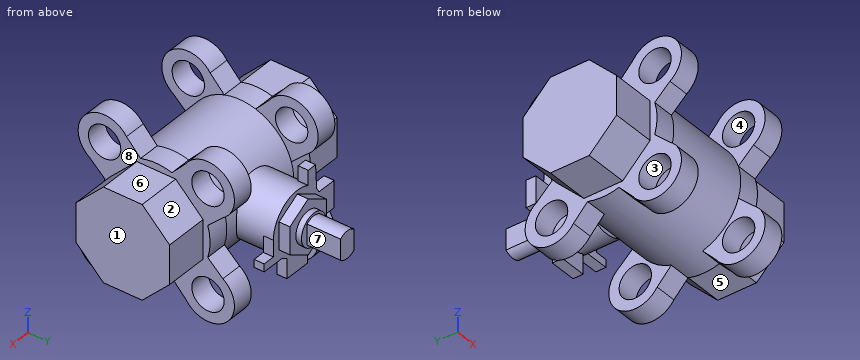
from build123d import *

# Parameters (mm, degrees)
SKETCH1_R            = 4.73075
BOSS_EXTRUDE2_DEPTH  = 6.35
BOSS_EXTRUDE3_DEPTH  = 12.7
SKETCH3_R            = 15.7226
BOSS_EXTRUDE4_DEPTH  = 25.4
SKETCH4_R            = 4.73075
BOSS_EXTRUDE5_DEPTH  = 6.35
BOSS_EXTRUDE6_DEPTH  = 12.7
SKETCH6_R            = 9.0805
BOSS_EXTRUDE8_DEPTH  = 12.8778
SKETCH8_W            = 7.8486
SKETCH8_H            = 8.0772
SKETCH8_W_2          = 8.0772
SKETCH8_H_2          = 7.8486
BOSS_EXTRUDE9_DEPTH  = 2.9464
BOSS_EXTRUDE10_DEPTH = 2.9464
BOSS_EXTRUDE11_DEPTH = 3.175
SKETCH12_R           = 4.6736
BOSS_EXTRUDE12_DEPTH = 1.651
BOSS_EXTRUDE13_DEPTH = 9.779


with BuildPart() as part:
    # Sketch1 → Boss-Extrude2 (new body)
    with BuildSketch(Plane(origin=(0, 0, 0), x_dir=(0, 0, -1), z_dir=(1, 0, 0))):
        with BuildLine():
            Line((-19.4818, 8.715375788), (-15.0368, 4.592907197))
            ThreePointArc((-15.0368, 4.592907197), (-15.7226, 0), (-15.0368, -4.592907197))
            Line((-15.0368, -4.592907197), (-19.4818, -8.715375788))
            ThreePointArc((-19.4818, -8.715375788), (-20.590956234, -20.590956234), (-8.715375788, -19.4818))
            Line((-8.715375788, -19.4818), (-4.592907197, -15.0368))
            ThreePointArc((-4.592907197, -15.0368), (0, -15.7226), (4.592907197, -15.0368))
            Line((4.592907197, -15.0368), (8.715375788, -19.4818))
            ThreePointArc((8.715375788, -19.4818), (20.590956234, -20.590956234), (19.4818, -8.715375788))
            Line((19.4818, -8.715375788), (15.0368, -4.592907197))
            ThreePointArc((15.0368, -4.592907197), (15.7226, 0), (15.0368, 4.592907197))
            Line((15.0368, 4.592907197), (19.4818, 8.715375788))
            ThreePointArc((19.4818, 8.715375788), (20.590956234, 20.590956234), (8.715375788, 19.4818))
            Line((8.715375788, 19.4818), (4.592907197, 15.0368))
            ThreePointArc((4.592907197, 15.0368), (0, 15.7226), (-4.592907197, 15.0368))
            Line((-4.592907197, 15.0368), (-8.715375788, 19.4818))
            ThreePointArc((-8.715375788, 19.4818), (-20.590956234, 20.590956234), (-19.4818, 8.715375788))
        make_face()
        with Locations((-15.113, 15.113)):
            Circle(SKETCH1_R, mode=Mode.SUBTRACT)
        with Locations((15.113, 15.113)):
            Circle(SKETCH1_R, mode=Mode.SUBTRACT)
        with Locations((15.113, -15.113)):
            Circle(SKETCH1_R, mode=Mode.SUBTRACT)
        with Locations((-15.113, -15.113)):
            Circle(SKETCH1_R, mode=Mode.SUBTRACT)
    extrude(amount=BOSS_EXTRUDE2_DEPTH)

    # Sketch2 → Boss-Extrude3 (add)
    with BuildSketch(Plane.ZY):
        Polygon((13.680992893, 5.666852803), (13.680992893, -5.666852803), (5.666852803, -13.680992893), (-5.666852803, -13.680992893), (-13.680992893, -5.666852803), (-13.680992893, 5.666852803), (-5.666852803, 13.680992893), (5.666852803, 13.680992893), align=None)
    extrude(amount=BOSS_EXTRUDE3_DEPTH)

    # Sketch3 → Boss-Extrude4 (add)
    with BuildSketch(Plane(origin=(6.35, 0, 0), x_dir=(0, 0, -1), z_dir=(1, 0, 0))):
        Circle(SKETCH3_R)
    extrude(amount=BOSS_EXTRUDE4_DEPTH)

    # Sketch4 → Boss-Extrude5 (add)
    with BuildSketch(Plane(origin=(31.75, 0, 0), x_dir=(0, 0, -1), z_dir=(1, 0, 0))):
        with BuildLine():
            Line((-19.4818, 8.715375788), (-15.0368, 4.592907197))
            ThreePointArc((-15.0368, 4.592907197), (-15.7226, 0), (-15.0368, -4.592907197))
            Line((-15.0368, -4.592907197), (-19.4818, -8.715375788))
            ThreePointArc((-19.4818, -8.715375788), (-20.590956234, -20.590956234), (-8.715375788, -19.4818))
            Line((-8.715375788, -19.4818), (-4.592907197, -15.0368))
            ThreePointArc((-4.592907197, -15.0368), (0, -15.7226), (4.592907197, -15.0368))
            Line((4.592907197, -15.0368), (8.715375788, -19.4818))
            ThreePointArc((8.715375788, -19.4818), (20.590956234, -20.590956234), (19.4818, -8.715375788))
            Line((19.4818, -8.715375788), (15.0368, -4.592907197))
            ThreePointArc((15.0368, -4.592907197), (15.7226, 0), (15.0368, 4.592907197))
            Line((15.0368, 4.592907197), (19.4818, 8.715375788))
            ThreePointArc((19.4818, 8.715375788), (20.590956234, 20.590956234), (8.715375788, 19.4818))
            Line((8.715375788, 19.4818), (4.592907197, 15.0368))
            ThreePointArc((4.592907197, 15.0368), (0, 15.7226), (-4.592907197, 15.0368))
            Line((-4.592907197, 15.0368), (-8.715375788, 19.4818))
            ThreePointArc((-8.715375788, 19.4818), (-20.590956234, 20.590956234), (-19.4818, 8.715375788))
        make_face()
        with Locations((-15.113, 15.113)):
            Circle(SKETCH4_R, mode=Mode.SUBTRACT)
        with Locations((15.113, 15.113)):
            Circle(SKETCH4_R, mode=Mode.SUBTRACT)
        with Locations((15.113, -15.113)):
            Circle(SKETCH4_R, mode=Mode.SUBTRACT)
        with Locations((-15.113, -15.113)):
            Circle(SKETCH4_R, mode=Mode.SUBTRACT)
    extrude(amount=BOSS_EXTRUDE5_DEPTH)

    # Sketch5 → Boss-Extrude6 (add)
    with BuildSketch(Plane(origin=(38.1, 0, 0), x_dir=(0, 0, -1), z_dir=(1, 0, 0))):
        Polygon((13.680992893, 5.666852803), (13.680992893, -5.666852803), (5.666852803, -13.680992893), (-5.666852803, -13.680992893), (-13.680992893, -5.666852803), (-13.680992893, 5.666852803), (-5.666852803, 13.680992893), (5.666852803, 13.680992893), align=None)
    extrude(amount=BOSS_EXTRUDE6_DEPTH)

    # Sketch6 → Boss-Extrude8 (add)
    with BuildSketch(Plane(origin=(0, 13.680992893, 0), x_dir=(1, 0, 0), z_dir=(0, 1, 0))):
        with Locations((19.05, 0.284018035)):
            Circle(SKETCH6_R)
    extrude(amount=BOSS_EXTRUDE8_DEPTH)

    # Sketch8 → Boss-Extrude9 (add)
    with BuildSketch(Plane(origin=(0, 26.558792893, 0), x_dir=(1, 0, 0), z_dir=(0, 1, 0))):
        with Locations((19.05, 10.202718035)):
            Rectangle(SKETCH8_W, SKETCH8_H)
        with Locations((9.1313, 0.284018035)):
            Rectangle(SKETCH8_W_2, SKETCH8_H_2)
    extrude(amount=-BOSS_EXTRUDE9_DEPTH)

    # Sketch10 → Boss-Extrude10 (add)
    with BuildSketch(Plane(origin=(0, 26.558792893, 0), x_dir=(1, 0, 0), z_dir=(0, 1, 0))):
        with BuildLine():
            Line((24.7523, 7.350789218), (31.6103, 7.350789218))
            Line((31.6103, 7.350789218), (31.6103, 5.064789218))
            Line((31.6103, 5.064789218), (28.1305, 5.064789218))
            Line((28.1305, 5.064789218), (28.1305, 0.284018035))
            ThreePointArc((28.1305, 0.284018035), (23.784459378, -7.464554392), (14.90647607, -7.795999892))
            Line((14.90647607, -7.795999892), (14.90647607, -12.140453608))
            Line((14.90647607, -12.140453608), (12.11247607, -12.140453608))
            Line((12.11247607, -12.140453608), (11.743935589, -5.108282316))
            ThreePointArc((11.743935589, -5.108282316), (12.769066077, 6.841864427), (24.7523, 7.350789218))
        make_face()
    extrude(amount=-BOSS_EXTRUDE10_DEPTH)

    # Sketch11 → Boss-Extrude11 (add)
    with BuildSketch(Plane(origin=(0, 26.558792893, 0), x_dir=(1, 0, 0), z_dir=(0, 1, 0))):
        Polygon((19.05, 8.285018035), (12.120930744, 4.284518035), (12.120930744, -3.716481965), (19.05, -7.716981965), (25.979069256, -3.716481965), (25.979069256, 4.284518035), align=None)
    extrude(amount=BOSS_EXTRUDE11_DEPTH)

    # Sketch12 → Boss-Extrude12 (add)
    with BuildSketch(Plane(origin=(0, 29.733792893, 0), x_dir=(1, 0, 0), z_dir=(0, 1, 0))):
        with Locations((19.05, 0.284018035)):
            Circle(SKETCH12_R)
    extrude(amount=BOSS_EXTRUDE12_DEPTH)

    # Sketch13 → Boss-Extrude13 (add)
    with BuildSketch(Plane(origin=(0, 31.384792893, 0), x_dir=(1, 0, 0), z_dir=(0, 1, 0))):
        with BuildLine():
            Line((16.51, 3.292068732), (16.51, -2.724032663))
            ThreePointArc((16.51, -2.724032663), (19.05, -3.652981965), (21.59, -2.724032663))
            Line((21.59, -2.724032663), (21.59, 3.292068732))
            ThreePointArc((21.59, 3.292068732), (19.05, 4.221018035), (16.51, 3.292068732))
        make_face()
    extrude(amount=BOSS_EXTRUDE13_DEPTH)


solid = part.part
Input: part model. Units: mm. Frame: model coordinates. Face numbers are marked on the shaded views. A direction names the side the tool comes from. Give positions to 0.01 mm unless a question says otherwise; leave off trailing zeros. Write each loop counter-clockwise with the first axis right and the second up, starting at its lowest first coordinate (ties: lowest second). Pieces come first, ordered by that corner, then holes.
Q1. Pull-direction query (Y, two-part tool) for the marked faces 1, 2, 3 and 4; classes: pulls with the +Y half, pulls with the -Y half, needs draft (parallel to the pull), parting line crosses it, or undercut.
Q2. Material intervals for probe 1 along Z at (x, y) = (2, 12.5); probe 2 along X at (y, z) = (38.5, 2); probe 3 along Z at (x, y) = (1, 20), sorted ascending.
Q3. Section A-A, the plane z = 18. State how many separate pieces and enclosed holes the cut face has, plus the area to 3 significant figures.
Q4. Set-up query: the marked faces 5, 6, 7 and 8. Return all of +Z, -Z, +X, -X, +Y, -Y with unobstructed straight access to the full face (end or side cutting, diameter ignored); none if empty.
Q5. First-contact query: P1, Ø5.5, axis at y = 16, z = 18, coming from the +X side; P2, Ø3.5, axis at x = -6, y = 2, coming from the -Z side; P3, Ø9, axis at y = 16.5, z = -12, coming from the -X side. Flat tips, straight axial feed; report the tip coordinate or a pass-through.
Q6. Section B-B, the plane x = 36. Output: boundary loops of the cut face in (y, z), plus the area to 3 significant figures.
Filled in:
1. face 1: needs draft
1. face 2: pulls with the +Y half
1. face 3: undercut
1. face 4: undercut
2. probe 1: z = -22.41 to -19.06, -11.17 to 11.17, 19.06 to 22.41
2. probe 2: x = 16.51 to 21.59
2. probe 3: z = -21.12 to -9.1, 9.1 to 21.12
3. separate pieces: 8
3. enclosed holes: 0
3. area: 190 mm2
4. face 5: -Z, +X, +Y, -Y
4. face 6: +Z, +X, +Y, -Y
4. face 7: +Z, -Z, +X, +Y
4. face 8: +X
5. P1: stops at x = 38.1
5. P2: stops at z = -13.68
5. P3: stops at x = 0
6. outline: (-19.48, -8.72) arc R7.75 ccw (long way) to (-8.72, -19.48) - (-4.59, -15.04) arc R15.72 ccw to (4.59, -15.04) - (8.72, -19.48) arc R7.75 ccw (long way) to (19.48, -8.72) - (15.04, -4.59) arc R15.72 ccw to (15.04, 4.59) - (19.48, 8.72) arc R7.75 ccw (long way) to (8.72, 19.48) - (4.59, 15.04) arc R15.72 ccw to (-4.59, 15.04) - (-8.72, 19.48) arc R7.75 ccw (long way) to (-19.48, 8.72) - (-15.04, 4.59) arc R15.72 ccw to (-15.04, -4.59) - close; hole circle Ø9.46 at (-15.11, -15.11); hole circle Ø9.46 at (-15.11, 15.11); hole circle Ø9.46 at (15.11, -15.11); hole circle Ø9.46 at (15.11, 15.11)
6. area: 1,250 mm2
